The listing builds one solid part. Answer for the finished solid, in the listing's coordinates (mm). Face numbers are marked on the shaded views. Round coordinates to 2 decimals unless told otherwise and drop trailing zeros. Write each loop counter-clockwise with the first axis right and the second up, starting at its lowest first coordinate (ties: lowest second). Pieces come first, ordered by that corner, then holes.
Autodesk Inventor part; units mm, degrees
ref_plane "YZ Plane" through (0, 0, 0) normal (1, 0, 0) x (0, 1, 0)
ref_plane "XZ Plane" through (0, 0, 0) normal (0, 1, 0) x (-1, 0, 0)
ref_plane "XY Plane" through (0, 0, 0) normal (0, 0, 1) x (1, 0, 0)
sketch "Эскиз1" plane through (0, 0, 0) normal (0, 0, 1) x (1, 0, 0)
  circle A0 centre (0, 0) radius 22
  line L0 (-4, 4) -> (4, 4)
  line L1 (4, 4) -> (4, -4)
  line L2 (4, -4) -> (-4, -4)
  line L3 (-4, -4) -> (-4, 4)
  line L4 (-4, 4) -> (4, -4) construction
  line L5 (4, 4) -> (-4, -4) construction
  circle A1 centre (0, 13.3333) radius 2
  circle A2 centre (-13.3333, 0) radius 2
  circle A3 centre (0, -13.3333) radius 2
  circle A4 centre (13.3333, 0) radius 2
  dimension "d0" = 44
  dimension "d1" = 8
  dimension "d2" = 8
  dimension "d3" = 4
  dimension "d5" = 13.3333
  dimension "d6" = 0
  dimension "d9" = 360
extrude "Выдавливание1" add sketch "Эскиз1" against normal blind 16 contours A0 | A1 | A2 | A3 | A4
hole "Отверстие1" at (13.3333, 0, 0) direction (0, 0, -1) diameter 4 end through all
hole "Отверстие2" at (-13.3333, 0, 0) direction (0, 0, -1) diameter 4 end through all
chamfer "Фаска1" distance 2 angle 45 1 edges at (-22, 0, -16)
ref_plane "РабПлоскость1" through (109, -4, 0) normal (-1, 0, 0) x (0, 0, 1)
sketch "Эскиз2" plane through (4, -4, 0) normal (-1, 0, 0) x (0, 0, 1)
  line L0 (0, -18) -> (0, 26)
  line L1 (-14, 26) -> (-14, -18)
  line L2 (-14, -18) -> (0, -18)
  line L3 (-14, 26) -> (0, 26)
sketch "Эскиз3" plane through (109, -4, 0) normal (-1, 0, 0) x (0, 0, 1)
  line L0 (0, -18) -> (0, 26) construction
  line L1 (-14, 26) -> (-14, -18) construction
  line L2 (0, -6.5) -> (-14, -6.5)
  line L3 (-14, -6.5) -> (-14, 14.5)
  line L4 (-14, 14.5) -> (0, 14.5)
  line L5 (0, 14.5) -> (0, -6.5)
  point P0 (0, 4)
  point P1 (0, 4)
  dimension "d53" = 21
  dimension "d54" = 14
sketch "Эскиз4" plane through (0, 0, 0) normal (0, 0, 1) x (1, 0, 0)
  circle A0 centre (0, 0) radius 22 construction
  line L0 (0, -22) -> (0, -4)
  arc A1 (0, 22) -> (109, 10.5) centre (90.7698, 360.0249) ccw
  arc A2 (109, -10.5) -> (0, -22) centre (90.7698, -360.0249) ccw
  line L1 (109, -10.5) -> (109, 10.5)
  circle A3 centre (13.3333, 0) radius 2
  line L2 (4, 4) -> (4, -4)
  line L3 (-4, 4) -> (4, 4)
  line L4 (4, -4) -> (-4, -4)
  line L5 (0, -4) -> (0, 4) construction
  line L6 (0, 4) -> (0, 22)
  line L7 (0, -43.0669) -> (0, 43.0669) construction
  arc A4 (109, -10.5) -> (109, 10.5) centre (109, 0) ccw
  point P0 (109, 10.5)
  point P1 (109, -10.5)
  dimension "d55" = 350
  dimension "d56" = 350
extrude "Выдавливание2" add sketch "Эскиз4" against normal blind 14
fillet "Сопряжение1" radius 50 2 edges at (10.4303, 19.3703, -7) (10.4303, -19.3703, -7)
equation "\"d53\" = 1.5 * d54"
equation "\"d56\" = d55"
properties part number "Ручной привод"
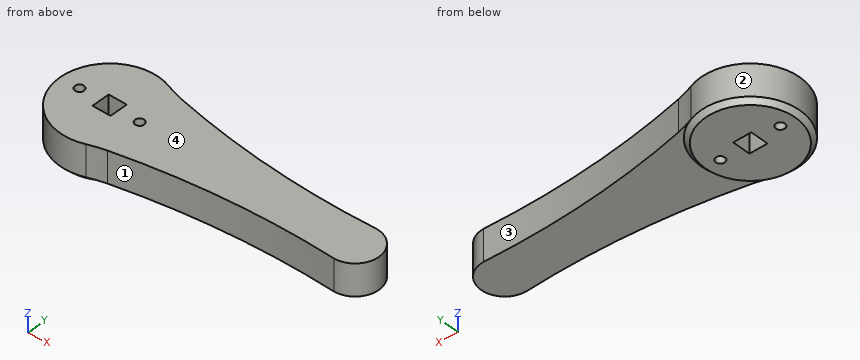
1. Given pin 1 (3 mm diameter, centred on y = 13.5, z = -4, fed in from -X); pin 2 (5 mm diameter, centred on x = -13.33, y = 0, fed in from +Z); pin 3 (4 mm diameter, centred on y = 8.5, z = -2.5, fed in from -X); pin 4 (8 mm diameter, centred on x = 74, z = -11.5, fed in from -Y), each flat-ended and moving along its own axis, determine where each tip first touches the part or whether it passes through.
Geometry says:
pin 1: stops at x = -18.44
pin 2: stops at z = 0
pin 3: stops at x = -21.02
pin 4: stops at y = -10.64
2. Section D-D on x = 34 is taken. Determine the outline of the cut face in (y, z), plus the area to 3 significant figures.
Geometry says:
outline: (-14.66, -14) - (14.66, -14) - (14.66, 0) - (-14.66, 0) - close
area: 410 mm2
3. For a pull along X with two mould halves and no side action, classify the marked faces 1, 2, 3 and 4 as released by +X, released by -X, zero draft, split by the parting line, or undercut.
Geometry says:
face 1: undercut
face 2: split by the parting line
face 3: undercut
face 4: zero draft
4. Section A-A on y = 0 is taken. Determine the outline of the cut face in (x, z), plus the area to 3 significant figures.
Geometry says:
outline: (-22, -14) - (-20, -16) - (-15.33, -16) - (-15.33, 0) - (-22, 0) - close; (-11.33, -16) - (-4, -16) - (-4, 0) - (-11.33, 0) - close; (4, -16) - (11.33, -16) - (11.33, 0) - (4, 0) - close; (15.33, -16) - (20, -16) - (22, -14) - (119.5, -14) - (119.5, 0) - (15.33, 0) - close
area: 1,810 mm2
5. Section C-C on z = -4 is taken. Give the number of separate pieces and of enclosed holes in the cut face, plus the area to 3 significant figures.
Geometry says:
separate pieces: 1
enclosed holes: 3
area: 3,770 mm2
6. Section B-B on x = 0 is taken. Determine the outline of the cut face in (y, z).
Geometry says:
outline: (-22, -14) - (-20, -16) - (-4, -16) - (-4, 0) - (-22, 0) - close; (4, -16) - (20, -16) - (22, -14) - (22, 0) - (4, 0) - close
7. Straight lines are drawn through the part: line 1 along X through (y, z) = (0, -10.5); line 2 along Z through (x, y) = (63, -9); line 3 along Y through (x, z) = (89.5, -4). For each, find the intervals that lie inside material, in ascending order.
Geometry says:
line 1: x = -22 to -15.33, -11.33 to -4, 4 to 11.33, 15.33 to 119.5
line 2: z = -14 to 0
line 3: y = -10.03 to 10.03
